For this review, take the finished solid that the model builds, in its own axes (mm). A direction names the side the tool comes from. Round coordinates to 2 decimals unless told otherwise and drop trailing zeros. Order: outer loops, then holes, each group sorted by start corner. A loop starts at its lowest first (then second) coordinate and runs counter-clockwise, first axis right, second up. Notation, with made-up numbers: (-12, 6) - (42, 6) arc R21 cw to (42, 24) - close; hole circle Ø2 at (-7, 34.25). An arc over 180 degrees is marked (long way). Write each question's results on one line, items separated by ' | '. Start each with the question number.
(1) For faces 1 (the flat face through (-1, 10, 10)), 2 (the flat face through (-106.89, 34.245, 9.86)), 3 (the flat face through (-29.9, -2.2, 5)), list the 3-axis set-ups (+Z, -Z, +X, -X, +Y, -Y) from which the entire face can be reached by the end or side of a thin tool; tool diameter is ignored.
(2) Take a section at C-C, the plane x = -8. Give the boundary of the cut face in (y, z), plus the area to 3 significant figures.
(3) Take a section at B-B, the plane z = 16.25. Give the boundary of the cut face in (x, y).
(4) For L1, parallel to Y at x = 15, z = 15.75; L2, parallel to X at y = 53, z = 4; L3, parallel to X at y = 74, z = 18.5, list the stretches that pass through material, from the lowest coordinate up. Write a range as from..to.
(5) Insertion check: pin 1 Ø8 at (x, y) = (31, -1) entering from -Z; pin 2 Ø6 at (y, z) = (51, 7) entering from -X; pin 3 Ø12 at (x, z) = (94.5, 17.5) entering from +Y; pin 4 Ø3 at (x, y) = (-31.5, 1.5) entering from -Z. Each pin has a flat end and moves straight along its axis. Give the tip position at first contact, or say it passes through.
(6) Take a section at D-D, the plane y = 55. Give the boundary of the cut face in (x, z).
(7) Draft analysis for pull direction Y (two halves, no side actions). For faces 4 (the cylindrical face through (-25, 0, 2)), 5 (the cylindrical face through (-61.851, -7.653, 10.14)), 6 (the flat face through (-93.75, 49.39, 9.86)), state which applies: pulls with the +Y half, pulls with the -Y half, needs draft (parallel to the pull), parting line crosses it, or undercut.
(8) Take a section at A-A, the plane y = 79. Give the boundary of the cut face in (x, z).
```python
from build123d import *

# Parameters (mm, degrees)
SKETCH_1_R          = 2
EXTRUDE_1_DEPTH     = 20
FILLET_1_R          = 10
FILLET_2_R          = 30
SKETCH_2_R          = 2.05
CUT_EXTRUDE_1_DEPTH = 50
SKETCH_3_R          = 5
CUT_EXTRUDE_2_DEPTH = 5
SKETCH_4_R          = 2.05
CUT_EXTRUDE_3_DEPTH = 29
SKETCH_5_R          = 2.15
CUT_EXTRUDE_4_DEPTH = 29


with BuildPart() as part:
    # 草图1 → 凸台-拉伸1 (new body)
    with BuildSketch(Plane.XY):
        Polygon((-143.355339059, 70.710678119), (-129.213203436, 84.852813742), (-54.360389693, 10), (54.360389693, 10), (129.213203436, 84.852813742), (143.355339059, 70.710678119), (62.644660941, -10), (-62.644660941, -10), align=None)
        with Locations((-122.142135624, 63.639610307)):
            Circle(SKETCH_1_R, mode=Mode.SUBTRACT)
        with Locations((122.142135624, 63.639610307)):
            Circle(SKETCH_1_R, mode=Mode.SUBTRACT)
    extrude(amount=EXTRUDE_1_DEPTH)

    # 圆角1
    fillet_1_edges = [part.edges().sort_by_distance(p)[0] for p in [
        (-54.360389693, 10, 10),
        (54.360389693, 10, 10),
    ]]
    fillet(fillet_1_edges, radius=FILLET_1_R)

    # 圆角2
    fillet_2_edges = [part.edges().sort_by_distance(p)[0] for p in [
        (62.644660941, -10, 10),
        (-62.644660941, -10, 10),
    ]]
    fillet(fillet_2_edges, radius=FILLET_2_R)

    # 草图2 → 切除-拉伸1 (cut)
    with BuildSketch(Plane.XY.offset(20)):
        with Locations((-30, 0)):
            Circle(SKETCH_2_R)
        with Locations((30, 0)):
            Circle(SKETCH_2_R)
    extrude(amount=-CUT_EXTRUDE_1_DEPTH, mode=Mode.SUBTRACT)

    # 草图3 → 切除-拉伸2 (cut)
    with BuildSketch(Plane(origin=(0, 0, 0), x_dir=(-1, 0, 0), z_dir=(0, 0, -1))):
        with Locations((-30, 0)):
            Circle(SKETCH_3_R)
        with Locations((30, 0)):
            Circle(SKETCH_3_R)
    extrude(amount=-CUT_EXTRUDE_2_DEPTH, mode=Mode.SUBTRACT)

    # 草图4 → 切除-拉伸3 (cut)
    with BuildSketch(Plane(origin=(0, 0, 0), x_dir=(-1, 0, 0), z_dir=(0, 0, -1))):
        with Locations((-20, 0)):
            Circle(SKETCH_4_R)
        with Locations((20, 0)):
            Circle(SKETCH_4_R)
    extrude(amount=-CUT_EXTRUDE_3_DEPTH, mode=Mode.SUBTRACT)

    # 草图5 → 切除-拉伸4 (cut)
    with BuildSketch(Plane.XZ.offset(10)):
        with Locations((-22, 10)):
            Circle(SKETCH_5_R)
        with Locations((22, 10)):
            Circle(SKETCH_5_R)
    extrude(amount=-CUT_EXTRUDE_4_DEPTH, mode=Mode.SUBTRACT)


solid = part.part
```
Results below:
1) face 1: +Z, -Z, +Y | face 2: +Z, -Z, -X, -Y | face 3: -Z
2) outline: (-10, 0) - (10, 0) - (10, 20) - (-10, 20) - close | area: 400 mm^2
3) outline: (-143.36, 70.71) - (-71.43, -1.21) arc R30 ccw to (-50.22, -10) - (50.22, -10) arc R30 ccw to (71.43, -1.21) - (143.36, 70.71) - (129.21, 84.85) - (57.29, 12.93) arc R10 cw to (50.22, 10) - (-50.22, 10) arc R10 cw to (-57.29, 12.93) - (-129.21, 84.85) - close; hole circle Ø4 at (-122.14, 63.64); hole circle Ø4.1 at (-30, 0); hole circle Ø4.1 at (-20, 0); hole circle Ø4.1 at (20, 0); hole circle Ø4.1 at (30, 0); hole circle Ø4 at (122.14, 63.64)
4) L1: y = -10..10 | L2: x = -125.64..-97.36, 97.36..125.64 | L3: x = -140.07..-118.36, 118.36..140.07
5) pin 1: stops at z = 0 | pin 2: stops at x = -126.64 | pin 3: stops at y = 56.14 | pin 4: stops at z = 5
6) outline: (-127.64, 0) - (-99.36, 0) - (-99.36, 20) - (-127.64, 20) - close; (99.36, 0) - (127.64, 0) - (127.64, 20) - (99.36, 20) - close
7) face 4: undercut | face 5: pulls with the -Y half | face 6: pulls with the +Y half
8) outline: (-135.07, 0) - (-123.36, 0) - (-123.36, 20) - (-135.07, 20) - close; (123.36, 0) - (135.07, 0) - (135.07, 20) - (123.36, 20) - close
